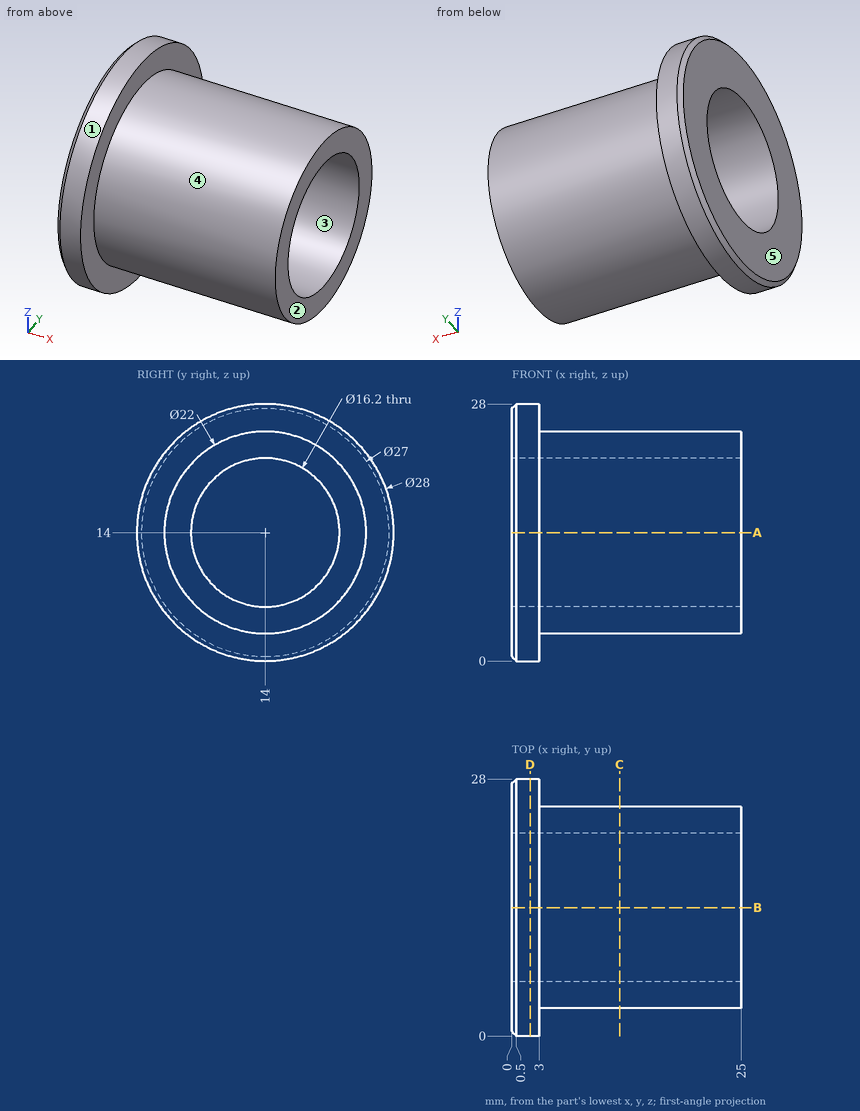
Check sheet for the drawn part. Datum: minimum x, y, z corner. Units: mm. A direction names the side the tool comes from. Coordinates: 2 decimals unless noted, no trailing zeros. Order: outer loops, then holes, each group sorted by start corner. A loop starts at its lowest first (then second) coordinate and runs counter-clockwise, first axis right, second up. Notation, with made-up numbers: M 52.5,50.25 L 75.5,50.25 A22 ccw 75.5,81.25 Z; hole C 44,78 d3. An arc over 180 degrees is marked long. One line per question, with ' | ' between items. Start each with the question number.
Item 1: Sectioned sample at A-A on z = 14. Record the cut outline in (x, y).
Item 2: Material ranges on line 1 (Y direction, x = 5.75, z = 14); line 2 (X direction, y = 25.25, z = 13.75); line 3 (Z direction, x = 8.75, y = 13), recorded low to high.
Item 3: Access from +Z, -Z, +X, -X, +Y, -Y to the whole of each face (thin tool, end or side, straight path). Record for the marked faces 4 and 5.
Item 4: Gauge pin test, flat ends, axial feed: P1, Ø5, axis at y = 25, z = 3.5, coming from the +X side; P2, Ø1, axis at x = 19, z = 14, coming from the -Y side; P3, Ø13, axis at y = 14, z = 14, coming from the -X side; P4, Ø4, axis at x = 9, z = 4, coming from the -Y side. Record the tip position at first contact, or that the pin passes through.
Item 5: Sectioned sample at C-C on x = 11.75. Record the cut outline in (y, z), and give its area (3 significant figures).
Item 6: Sectioned sample at D-D on x = 2. Record the cut outline in (y, z), and give its area (3 significant figures).
Item 7: Mould release check, pull along Z, two halves, no side actions. Record for the marked faces 1, 2 and 3: pulls with the +Z half, pulls with the -Z half, needs draft (parallel to the pull), parting line crosses it, or undercut.
Answer below:
1) outline: M 0,0.5 L 0.5,0 L 3,0 L 3,3 L 25,3 L 25,5.9 L 0,5.9 Z; M 0,22.1 L 25,22.1 L 25,25 L 3,25 L 3,28 L 0.5,28 L 0,27.5 Z
2) line 1: y = 3 to 5.9, 22.1 to 25 | line 2: x = 0 to 3 | line 3: z = 3.05 to 5.96, 22.04 to 24.95
3) face 4: +X | face 5: +Z, -Z, -X, +Y, -Y
4) P1: stops at x = 3 | P2: stops at y = 3 | P3: passes through | P4: stops at y = 6.45
5) outline: C 14,14 d22; hole C 14,14 d16.2 | area: 174 mm^2
6) outline: C 14,14 d28; hole C 14,14 d16.2 | area: 410 mm^2
7) face 1: parting line crosses it | face 2: needs draft | face 3: undercut
